```python
from build123d import *

# Parameters (mm, degrees)
SKETCH1_W           = 10
SKETCH1_H           = 10
BOSS_EXTRUDE1_DEPTH = 75
SKETCH3_W           = 7.5
SKETCH3_H           = 4.25
CUT_EXTRUDE1_DEPTH  = 7.5
SKETCH4_W           = 2
SKETCH4_H           = 5.5
CUT_EXTRUDE2_DEPTH  = 73.25
SKETCH5_W           = 10
SKETCH5_H           = 10
BOSS_EXTRUDE2_DEPTH = 3.25
BOSS_EXTRUDE3_REACH = 78.322
SKETCH6_W           = 1
SKETCH6_H           = 1.9
SKETCH6_H_2         = 2
SKETCH7_R           = 2.175
CUT_EXTRUDE3_DEPTH  = 3
SKETCH8_W           = 8.5
SKETCH8_H           = 1.5
CUT_EXTRUDE4_DEPTH  = 80.517686712
FILLET1_SIZE        = 0.9


with BuildPart() as part:
    # Sketch1 → Boss-Extrude1 (new body)
    with BuildSketch(Plane(origin=(0, 0, 0), x_dir=(1, 0, 0), z_dir=(0, 1, 0))):
        with Locations((5, 5)):
            Rectangle(SKETCH1_W, SKETCH1_H)
    extrude(amount=BOSS_EXTRUDE1_DEPTH)

    # Sketch3 → Cut-Extrude1 (cut)
    with BuildSketch(Plane(origin=(0, 0, -10), x_dir=(-1, 0, 0), z_dir=(0, 0, -1))):
        with Locations((-6.25, 71.125)):
            Rectangle(SKETCH3_W, SKETCH3_H)
    extrude(amount=-CUT_EXTRUDE1_DEPTH, mode=Mode.SUBTRACT)

    # Sketch4 → Cut-Extrude2 (cut)
    with BuildSketch(Plane.XZ):
        Polygon((10, -2.5), (2.5, -2.5), (2.5, -4.5), (4.5, -4.5), (10, -4.5), align=None)
        with Locations((3.5, -7.25)):
            Rectangle(SKETCH4_W, SKETCH4_H)
    extrude(amount=-CUT_EXTRUDE2_DEPTH, mode=Mode.SUBTRACT)


with BuildPart() as cut_extrude2_piece_1:
    # of the separate pieces the step leaves, piece 1, a body of its own (cut_extrude2_pieces)
    add(part.part.solids().sort_by_distance((0, 0, 0))[0])



with BuildPart() as cut_extrude2_piece_2:
    # of the separate pieces the step leaves, piece 2, a body of its own (cut_extrude2_pieces)
    add(part.part.solids().sort_by_distance((10, 0, -4.5))[0])


with BuildPart() as cut_extrude2_piece_1_1:
    add(cut_extrude2_piece_1.part)

    add(cut_extrude2_piece_2.part)  # Boss-Extrude2 merges Cut-Extrude2 piece 2
    # Sketch5 → Boss-Extrude2 (add)
    with BuildSketch(Plane.XZ):
        with Locations((5, -5)):
            Rectangle(SKETCH5_W, SKETCH5_H)
    extrude(amount=BOSS_EXTRUDE2_DEPTH)

    # Boss-Extrude3: up to this face of the body (flat: up to its plane)
    boss_extrude3_end = Plane(cut_extrude2_piece_1_1.part.faces().sort_by_distance((6.25, 73.25, -6.25))[0])
    # Sketch6 → Boss-Extrude3 (add, up to the picked face)
    with BuildSketch(Plane(origin=(0, 0, 0), x_dir=(1, 0, 0), z_dir=(0, 1, 0)), mode=Mode.PRIVATE) as boss_extrude3_sk1:
        Polygon((3.5, 4.5), (3.5, 2.5), (6.4, 2.5), (6.4, 4.5), (4.5, 4.5), align=None)
    boss_extrude3_tool1 = split(extrude(boss_extrude3_sk1.sketch, amount=BOSS_EXTRUDE3_REACH, mode=Mode.PRIVATE), bisect_by=boss_extrude3_end, keep=Keep.BOTH, mode=Mode.PRIVATE)
    # Sketch6 → Boss-Extrude3 (add, up to the picked face)
    with BuildSketch(Plane(origin=(0, 0, 0), x_dir=(1, 0, 0), z_dir=(0, 1, 0)), mode=Mode.PRIVATE) as boss_extrude3_sk2:
        with Locations((4, 5.45)):
            Rectangle(SKETCH6_W, SKETCH6_H)
    boss_extrude3_tool2 = split(extrude(boss_extrude3_sk2.sketch, amount=BOSS_EXTRUDE3_REACH, mode=Mode.PRIVATE), bisect_by=boss_extrude3_end, keep=Keep.BOTH, mode=Mode.PRIVATE)
    # Sketch6 → Boss-Extrude3 (add, up to the picked face)
    with BuildSketch(Plane(origin=(0, 0, 0), x_dir=(1, 0, 0), z_dir=(0, 1, 0)), mode=Mode.PRIVATE) as boss_extrude3_sk3:
        with Locations((3, 5.45)):
            Rectangle(SKETCH6_W, SKETCH6_H)
    boss_extrude3_tool3 = split(extrude(boss_extrude3_sk3.sketch, amount=BOSS_EXTRUDE3_REACH, mode=Mode.PRIVATE), bisect_by=boss_extrude3_end, keep=Keep.BOTH, mode=Mode.PRIVATE)
    # Sketch6 → Boss-Extrude3 (add, up to the picked face)
    with BuildSketch(Plane(origin=(0, 0, 0), x_dir=(1, 0, 0), z_dir=(0, 1, 0)), mode=Mode.PRIVATE) as boss_extrude3_sk4:
        with Locations((3, 3.5)):
            Rectangle(SKETCH6_W, SKETCH6_H_2)
    boss_extrude3_tool4 = split(extrude(boss_extrude3_sk4.sketch, amount=BOSS_EXTRUDE3_REACH, mode=Mode.PRIVATE), bisect_by=boss_extrude3_end, keep=Keep.BOTH, mode=Mode.PRIVATE)
    add(boss_extrude3_tool1.solids().sort_by(Axis((4.95, 0, -3.5), (0, 1, 0)))[0])
    add(boss_extrude3_tool2.solids().sort_by(Axis((4, 0, -5.45), (0, 1, 0)))[0])
    add(boss_extrude3_tool3.solids().sort_by(Axis((3, 0, -5.45), (0, 1, 0)))[0])
    add(boss_extrude3_tool4.solids().sort_by(Axis((3, 0, -3.5), (0, 1, 0)))[0])

    # Sketch7 → Cut-Extrude3 (cut)
    with BuildSketch(Plane.XZ.offset(3.25)):
        with Locations(Location((5, -5, 0), (0, 0, 270))):
            Circle(SKETCH7_R)
    extrude(amount=-CUT_EXTRUDE3_DEPTH, mode=Mode.SUBTRACT)

    # Sketch8 → Cut-Extrude4 (cut, through all)
    with BuildSketch(Plane(origin=(0, 75, 0), x_dir=(1, 0, 0), z_dir=(0, 1, 0))):
        Polygon((1.5, 10), (0, 10), (0, 0), (1.5, 0), (1.5, 1.5), align=None)
        with Locations((5.75, 0.75)):
            Rectangle(SKETCH8_W, SKETCH8_H)
    extrude(amount=-CUT_EXTRUDE4_DEPTH, mode=Mode.SUBTRACT)

    # Fillet1
    # a fillet whose section is not a circle: 0.9 mm, written as the material it takes off along each edge
    with BuildSketch(Plane(origin=(10, 77.25, -1.5), x_dir=(0, 0, -1), z_dir=(0, -1, 0)), Plane(origin=(1.5, 77.25, -1.5), x_dir=(1, 0, 0), z_dir=(0, -1, 0))) as fillet1_piece_1:
        with BuildLine():
            Bezier((FILLET1_SIZE, 0), (0, 0), (0, -FILLET1_SIZE), weights=[1, 0.052631579, 1])
            Line((0, -FILLET1_SIZE), (0, 0))
            Line((0, 0), (FILLET1_SIZE, 0))
        make_face()
    extrude(amount=82.75, mode=Mode.SUBTRACT)
    with BuildSketch(Plane(origin=(1.5, 77.25, -10), x_dir=(1, 0, 0), z_dir=(0, -1, 0))) as fillet1_piece_2:
        with BuildLine():
            Bezier((FILLET1_SIZE, 0), (0, 0), (0, FILLET1_SIZE), weights=[1, 0.052631579, 1])
            Line((0, FILLET1_SIZE), (0, 0))
            Line((0, 0), (FILLET1_SIZE, 0))
        make_face()
    extrude(amount=82.75, mode=Mode.SUBTRACT)


solid = cut_extrude2_piece_1_1.part
```
Verification items for the finished model (mm, model axes). A direction names the side the tool comes from. Give positions to 0.01 mm unless a question says otherwise; leave off trailing zeros. Return JSON: item names as keys, results as strings.
1) Mould release check, pull along Z, two halves, no side actions. Record for faces 5 (the flat face through (8, 36, -10)), 6 (the flat face through (6, 36, -1.5)), 7 (the flat face through (7, 73.25, -7)), 8 (the flat face through (6.4, 36, -3)): released by +Z, released by -Z, zero draft, split by the parting line, or undercut.
Findings:
{"face 5": "released by -Z", "face 6": "released by +Z", "face 7": "zero draft", "face 8": "undercut"}
2) Tool access check on faces 1 (the flat face through (7, 69, -7)), 2 (the flat face through (8, 36, -2.5)), 3 (the flat face through (10, 36, -7)), 4 (the flat face through (4.5, 34, -8)). Record the directions out of +Z, -Z, +X, -X, +Y, -Y that give a thin tool (end or side, any length) a straight path to the whole face; none if there is none.
Findings:
{"face 1": "-Z, +X", "face 2": "+X", "face 3": "+Z, -Z, +X, +Y, -Y", "face 4": "-Z"}
3) Material ranges on L1, parallel to X at y = -1.6, z = -5 (3 decimals); L2, parallel to Y at x = 7.5, z = -7.5; L3, parallel to Y at x = 8, z = -3.75, recorded low to high. Write a range as [from, to].
Findings:
{"L1": "x = [1.5, 2.825], [7.175, 10]", "L2": "y = [-3.25, 69], [73.25, 75]", "L3": "y = [-3.25, 0], [73.25, 75]"}
4) Gauge pin test, flat ends, axial feed: P1, Ø0.6, axis at x = 3.5, y = 21, coming from the -Z side; P2, Ø0.6, axis at y = 71.5, z = -6, coming from the +X side; P3, Ø1.3, axis at x = 5.5, z = -6, coming from the -Y side. Record the tip position at first contact, or that the pin passes through.
Findings:
{"P1": "stops at z = -6.4", "P2": "stops at x = 4.5", "P3": "stops at y = -0.25"}
